Build history of the part. All positions in model axes, mm. A direction names the side the tool comes from. Coordinates: 2 decimals unless noted, no trailing zeros. Write each loop counter-clockwise with the first axis right and the second up, starting at its lowest first coordinate (ties: lowest second). Pieces come first, ordered by that corner, then holes.
```python
from build123d import *

# Parameters (mm, degrees)
F0_W     = 6.35
F0_H     = 31.75
F1_DEPTH = 3.175
F2_R     = 5.08
F3_R     = 1.27
F4_DEPTH = 53.34
F5_W     = 21.59
F5_H     = 7.036624
F6_DEPTH = 25.4


with BuildPart() as f1:
    # F0 (on Front) → F1 (new body, symmetric)
    with BuildSketch(Plane.XZ):
        with Locations((0, 25.4)):
            Rectangle(F0_W, F0_H)
        Polygon((3.175, 9.525), (-3.175, 9.525), (-12.7, 9.525), (-12.7, -9.525), (12.7, -9.525), (12.7, 9.525), align=None)
    extrude(amount=F1_DEPTH, both=True)

    # F2
    f2_edges = [f1.edges().sort_by_distance(p)[0] for p in [
        (0, 3.175, 41.275),
    ]]
    fillet(f2_edges, radius=F2_R)

    # F3 (on face) → F4 (cut)
    with BuildSketch(Plane.YZ.offset(3.175)):
        with Locations((0, 36.86247)):
            Circle(F3_R)
    extrude(amount=-F4_DEPTH, mode=Mode.SUBTRACT)

    # F5 (on face) → F6 (cut, symmetric)
    with BuildSketch(Plane.XZ.offset(3.175)):
        Rectangle(F5_W, F5_H)
    extrude(amount=F6_DEPTH, both=True, mode=Mode.SUBTRACT)


solid = f1.part
```
1. 3-axis set-ups, long thin cutter, end or side, ignore diameter. For faces 1 (the face through (-8, 0, 9.525)), 2 (the face through (3.175, 0, 25)), 3 (the face through (0, 0, 3.518)): which of +Z, -Z, +X, -X, +Y, -Y reach the whole face in a straight line?
Computed values:
face 1: +Z, -X, +Y, -Y
face 2: +Z, +X, +Y, -Y
face 3: +Y, -Y
2. Saw through at A-A on x = -4.25. List the corners of the cut face in (y, z) (3 decimals).
Computed values:
outline: (-3.175, -9.525) - (3.175, -9.525) - (3.175, -3.518) - (-3.175, -3.518) - close; (-3.175, 3.518) - (3.175, 3.518) - (3.175, 9.525) - (-3.175, 9.525) - close
3. Mould opens along Y. For faces 4 (the face through (0.04, -0.17, 38.12)), 5 (the face through (0, 3.175, 9)), 6 (the face through (10.795, 0, 0)) say: +Y half, -Y half, draft (parallel to the pull), parting line (faces both ways), or undercut.
Computed values:
face 4: undercut
face 5: +Y half
face 6: draft
4. Probe line 1 along X through (y, z) = (0, -2) (3 decimals); line 2 along Z through (x, y) = (-1.5, 0) (3 decimals); line 3 along Z through (x, y) = (6.5, -1) (3 decimals). List the from-to ranges inside material, lowest first.
Computed values:
line 1: x = -12.7 to -10.795, 10.795 to 12.7
line 2: z = -9.525 to -3.518, 3.518 to 35.592, 38.132 to 40.904
line 3: z = -9.525 to -3.518, 3.518 to 9.525
5. Saw through at C-C on x = 1.5. List the corners of the cut face in (y, z) (3 decimals).
Computed values:
outline: (-3.175, -9.525) - (3.175, -9.525) - (3.175, -3.518) - (-3.175, -3.518) - close; (-3.175, 3.518) - (3.175, 3.518) - (3.175, 36.195) arc R5.08 ccw to (-1.905, 41.275) - (-3.175, 41.275) - close; hole circle Ø2.54 at (0, 36.862)
6. Saw through at B-B on z = 2. List the corners of the cut face in (x, y) (3 decimals).
Computed values:
outline: (-12.7, -3.175) - (-10.795, -3.175) - (-10.795, 3.175) - (-12.7, 3.175) - close; (10.795, -3.175) - (12.7, -3.175) - (12.7, 3.175) - (10.795, 3.175) - close
7. Flat gauge pins, fed straight in: pin 1 (1 mm diameter, centred on x = -6, y = -1, fed in from +Z) (3 decimals); pin 2 (1.9 mm diameter, centred on x = 2.5, y = 1, fed in from +Z); pin 3 (3 mm diameter, centred on y = 1, z = 23, fed in from +X) (3 decimals). Where does each tip first touch, or does it go through?
Computed values:
pin 1: stops at z = 9.525
pin 2: stops at z = 40.88
pin 3: stops at x = 3.175
